Design review of the part shown in the three views and the two pictorial views. Dimensions are in mm from the part's minimum x, y and z. Coordinates: 2 decimals unless noted, no trailing zeros. Loops run counter-clockwise (first coordinate to the right, second up) from the corner with the lowest first, then second, coordinate; pieces in that order, holes last. Notation, with made-up numbers: M -19.5,14.5 L 31.5,14.5 A33 ccw 31.5,50.5 Z; hole C 72.25,57 d5. An arc over 180 degrees is marked long. Write item = value, one per line. Start each with the question number.
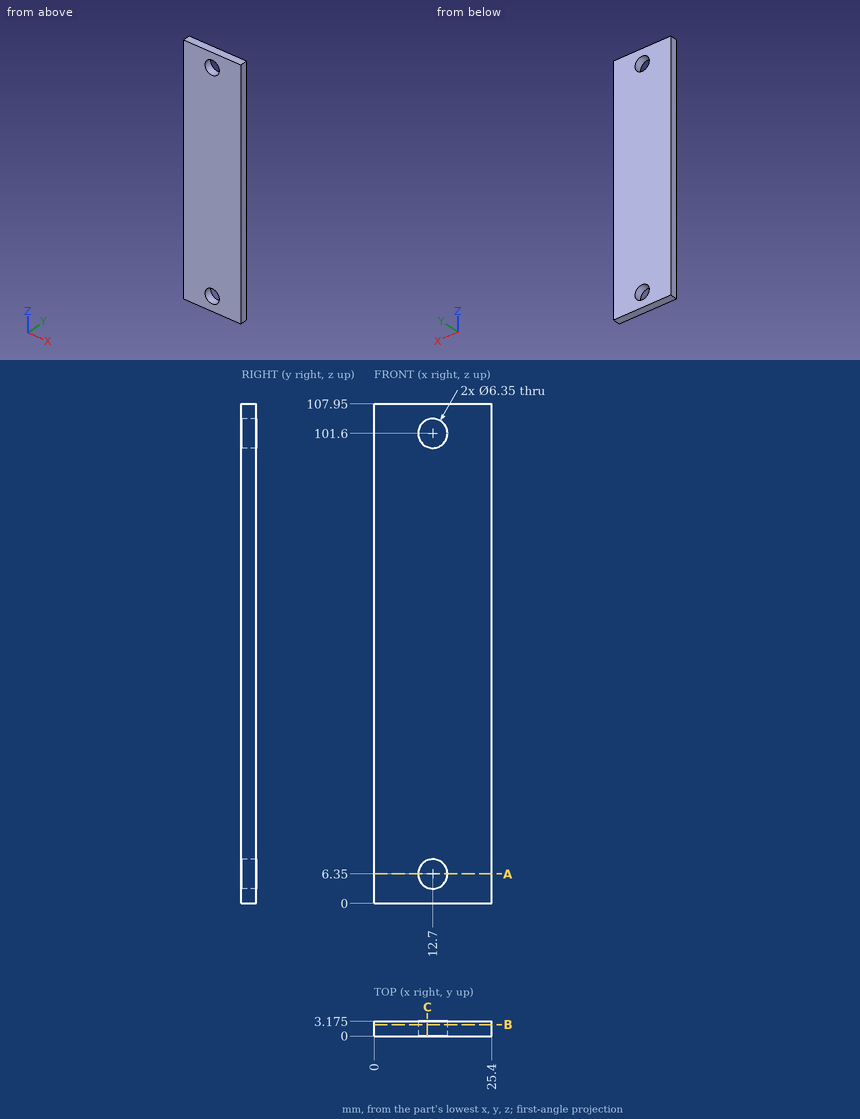
(1) Take a section at B-B (y = 2.45). State the section outline as (x, z) points (3 decimals), plus the area to 3 significant figures.
(2) Take a section at A-A (z = 6.35). State the section outline as (x, y) points (3 decimals), plus the area to 3 significant figures.
(3) To check wall thickness, follow L1, parallel to Z at x = 12.7, y = 2.35 (3 decimals); L2, parallel to Z at x = 11.25, y = 0.9; L3, parallel to X at y = 1.1, z = 103.5. State the ranges of each line that lie inside material, in increasing order.
(4) Insertion check: pin 1 (5.5 mm diameter, centred on x = 12.7, z = 101.6, fed in from -Y). The pin has a flat end and moves straight along its axis. Give the tip position at first contact, or say it passes through.
(5) Take a section at C-C (x = 11.5). Give the number of separate pieces and of enclosed holes in the cut face, plus the area to 3 significant figures.
Results list:
q1.outline = M 0,0 L 25.4,0 L 25.4,107.95 L 0,107.95 Z; hole C 12.7,6.35 d6.35; hole C 12.7,101.6 d6.35
q1.area = 2,680 mm^2
q2.outline = M 0,0 L 9.525,0 L 9.525,3.175 L 0,3.175 Z; M 15.875,0 L 25.4,0 L 25.4,3.175 L 15.875,3.175 Z
q2.area = 60.5 mm^2
q3.L1 = 0 to 3.175, 9.525 to 98.425, 104.775 to 107.95
q3.L2 = 0 to 3.53, 9.17 to 98.78, 104.42 to 107.95
q3.L3 = 0 to 10.16, 15.24 to 25.4
q4.pin_1 = through
q5.separate_pieces = 3
q5.enclosed_holes = 0
q5.area = 305 mm^2
